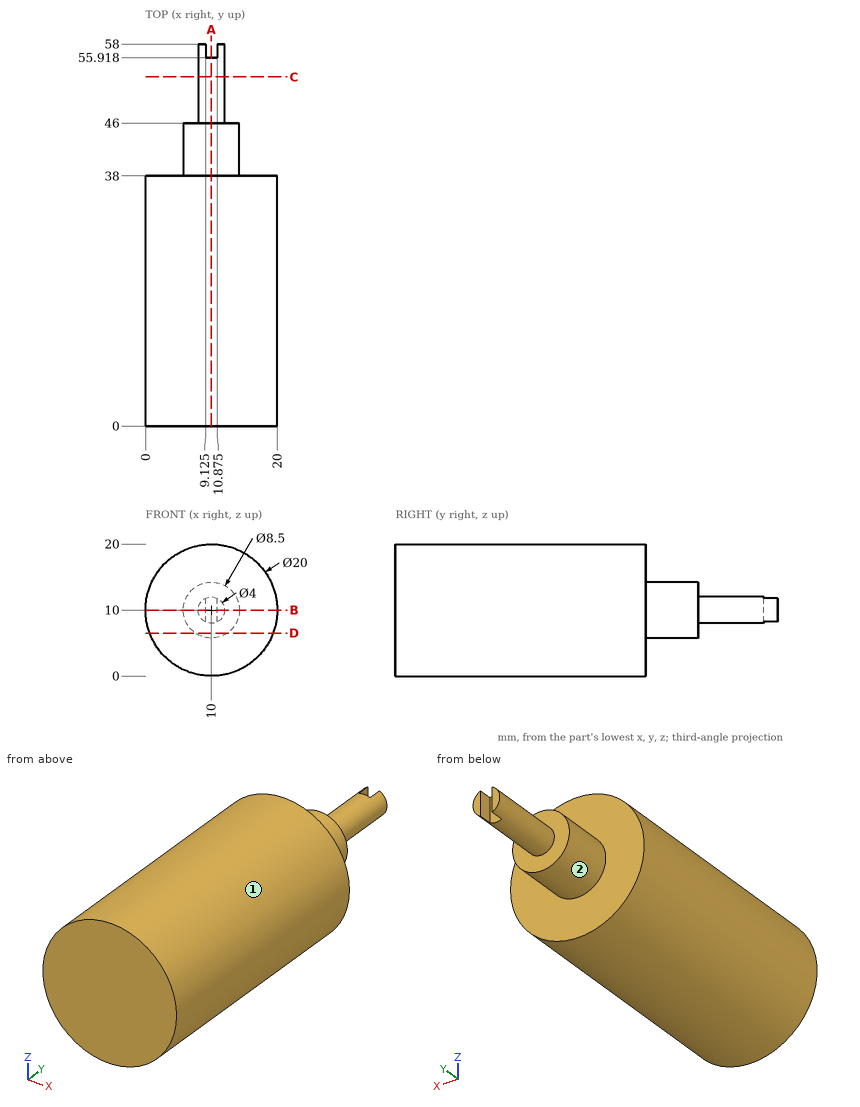
Study the drawing (mm; zero at the part's minimum x, y, z) and answer. A direction names the side the tool comes from. Give positions to 0.01 mm unless a question says otherwise; leave off trailing zeros. Write each loop counter-clockwise with the first axis right and the second up, starting at its lowest first coordinate (ties: lowest second). Pieces come first, ordered by that corner, then holes.
Item 1: Section A-A, the plane x = 10 is taken. Write down the section's boundary in (y, z), plus the area to 3 significant figures.
Item 2: Section D-D, the plane z = 6.5 is taken. Write down the section's boundary in (x, y).
Item 3: Find the intervals of material crossed by line 1 along Y through (x, z) = (18.5, 8.5); line 2 along Z through (x, y) = (9.75, 20); line 3 along Y through (x, z) = (7, 9.75), in increasing order.
Item 4: Which of the six approach directions +Z, -Z, +X, -X, +Y, -Y give full straight-line access (tool end or side, diameter ignored) to the marked faces 1 and 2?
Item 5: Section B-B, the plane z = 10 is taken. Write down the section's boundary in (x, y) (3 decimals).
Item 6: Section C-C, the plane y = 53 is taken. Write down the section's boundary in (x, z).
Item 7: Flat-ended cylindrical pins translate along their axes: P1, Ø1.7, axis at y = 57, z = 10.5, coming from the -X side; P2, Ø2, axis at x = 7.5, y = 26, coming from the +Z side; P3, Ø2.5, axis at y = 56.5, z = 10.5, coming from the +X side; P4, Ø8, axis at x = 3, z = 11, coming from the -Y side. Find the tip coordinate at first contact, or state that the pin passes through.
Completed:
1. outline: (0, 0) - (38, 0) - (38, 5.75) - (46, 5.75) - (46, 8) - (55.92, 8) - (55.92, 12) - (46, 12) - (46, 14.25) - (38, 14.25) - (38, 20) - (0, 20) - close
1. area: 868 mm2
2. outline: (0.63, 0) - (19.37, 0) - (19.37, 38) - (12.41, 38) - (12.41, 46) - (7.59, 46) - (7.59, 38) - (0.63, 38) - close
3. line 1: y = 0 to 38
3. line 2: z = 0 to 20
3. line 3: y = 0 to 46
4. face 1: +Y, -Y
4. face 2: +Y
5. outline: (0, 0) - (20, 0) - (20, 38) - (14.25, 38) - (14.25, 46) - (12, 46) - (12, 58) - (10.875, 58) - (10.875, 55.918) - (9.125, 55.918) - (9.125, 58) - (8, 58) - (8, 46) - (5.75, 46) - (5.75, 38) - (0, 38) - close
6. outline: circle Ø4 at (10, 10)
7. P1: stops at x = 8
7. P2: stops at z = 19.89
7. P3: stops at x = 12
7. P4: stops at y = 0
